Verification items for the finished model (mm, model axes). Coordinates: 2 decimals unless noted, no trailing zeros. Loops run counter-clockwise (first coordinate to the right, second up) from the corner with the lowest first, then second, coordinate; pieces in that order, holes last. Notation, with made-up numbers: M 57,71 L 97,71 A17 ccw 97,87 Z; hole C 16,38 d5. An arc over 180 degrees is marked long. Write item = value, one per line. Start each with the question number.
```python
from build123d import *

# Parameters (mm, degrees)
F0_W     = 57.15
F0_H     = 55.88
F0_R     = 3.175
F0_R_2   = 1.905
F1_DEPTH = 3.81
F2_R     = 2.54
F3_R     = 1.27


with BuildPart() as f1:
    # F0 (on Top) → F1 (new body)
    with BuildSketch(Plane.XY):
        with Locations((24.765, 15.24)):
            Rectangle(F0_W, F0_H)
        with Locations((1.524, -6.35)):
            Circle(F0_R, mode=Mode.SUBTRACT)
        Circle(F0_R_2, mode=Mode.SUBTRACT)
        with Locations((48.26, -6.35)):
            Circle(F0_R, mode=Mode.SUBTRACT)
        with Locations((49.53, 0)):
            Circle(F0_R_2, mode=Mode.SUBTRACT)
        with Locations((0, 36.195)):
            Circle(F0_R_2, mode=Mode.SUBTRACT)
        Polygon((4.773997, -1.905), (1.905, 4.693742), (1.905, 32.801047), (5.652351, 39.363042), (45.657352, 39.363042), (49.53, 36.195), (49.53, 31.363741), (48.212558, 30.086137), (48.212558, 4.29449), (44.938698, -1.905), align=None, mode=Mode.SUBTRACT)
    extrude(amount=F1_DEPTH)

    # F2
    f2_edges = [f1.edges().sort_by_distance(p)[0] for p in [
        (-3.81, -12.7, 1.905),
        (-3.81, 43.18, 1.905),
        (53.34, -12.7, 1.905),
        (53.34, 43.18, 1.905),
        (1.905, 32.801047, 1.905),
        (5.652351, 39.363042, 1.905),
        (1.905, 4.693742, 1.905),
        (4.773997, -1.905, 1.905),
        (45.657352, 39.363042, 1.905),
        (49.53, 36.195, 1.905),
        (48.212558, 30.086137, 1.905),
        (48.212558, 4.29449, 1.905),
        (44.938698, -1.905, 1.905),
    ]]
    fillet(f2_edges, radius=F2_R)

    # F3
    f3_edges = [f1.edges().sort_by_distance(p)[0] for p in [
        (49.53, 31.363741, 1.905),
    ]]
    fillet(f3_edges, radius=F3_R)


solid = f1.part
```
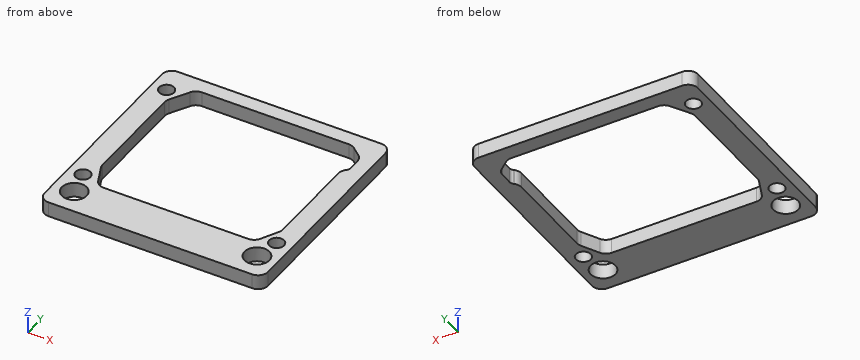
Q1. Sectioned sample at D-D on z = 2.1. Count the separate pieces of the cut face and the enclosed holes in it, plus the area to 3 significant figures.
Q2. Sectioned sample at C-C on y = -6.35. Record the cut outline in (x, z) (3 decimals), plus the area to 3 significant figures.
Q3. Sectioned sample at B-B on x = 24. Record the cut outline in (y, z) (3 decimals), plus the area to 3 significant figures.
Q4. Scan lines: L1, parallel to X at y = 11.5, z = 1.4 (3 decimals); L2, parallel to Y at x = 43.5, z = 0.8; L3, parallel to Y at x = 44.5, z = 1.6. Record each from-to range of solid material in increasing order. Write a range as [from, to].
Q5. Sectioned sample at A-A on y = 16. Record the cut outline in (x, z) (3 decimals), plus the area to 3 significant figures.
Q6. Gauge pin test, flat end, axial feed: pin 1 (2.5 mm diameter, centred on x = 0, y = 36.195, fed in from -Z). Record the tip position at first contact, or that the pin passes through.
Solutions:
q1.separate_pieces = 1
q1.enclosed_holes = 6
q1.area = 1,210 mm²
q2.outline = M -3.81,0 L -1.651,0 L -1.651,3.81 L -3.81,3.81 Z; M 4.699,0 L 45.085,0 L 45.085,3.81 L 4.699,3.81 Z; M 51.435,0 L 53.34,0 L 53.34,3.81 L 51.435,3.81 Z
q2.area = 169 mm²
q3.outline = M -12.7,0 L -1.905,0 L -1.905,3.81 L -12.7,3.81 Z; M 39.363,0 L 43.18,0 L 43.18,3.81 L 39.363,3.81 Z
q3.area = 55.7 mm²
q4.L1 = [-3.81, 1.905], [48.213, 53.34]
q4.L2 = [-12.7, -1.9], [39.36, 43.18]
q4.L3 = [-12.7, -1.66], [39.36, 43.18]
q5.outline = M -3.81,0 L 1.905,0 L 1.905,3.81 L -3.81,3.81 Z; M 48.213,0 L 53.34,0 L 53.34,3.81 L 48.213,3.81 Z
q5.area = 41.3 mm²
q6.pin_1 = through
